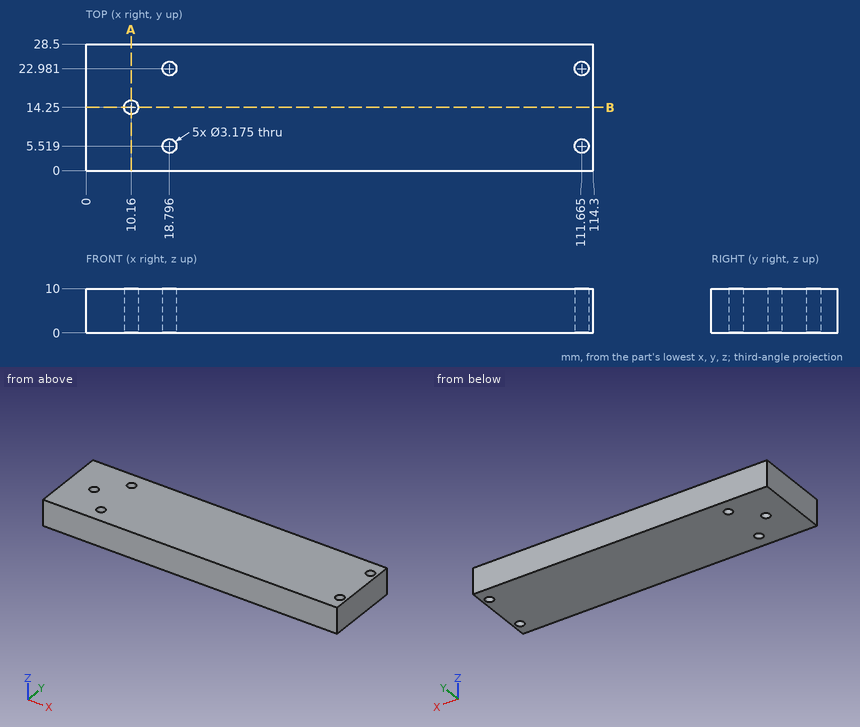
Geometry: see drawing. Coordinates: mm, zero at the bounding-box minimum. Give positions to 0.01 mm unless a question says otherwise; leave off trailing zeros. Order: outer loops, then holes, each group sorted by start corner. A loop starts at its lowest first (then second) coordinate and runs counter-clockwise, first axis right, second up. Notation, with made-up numbers: M -38,-23.5 L -14,-23.5 A19 cw -14,7.5 Z; hole C 60,61 d9. An arc over 180 degrees is marked long. Answer as a JSON object with one key per item and string values.
1. Cut plane B-B, the plane y = 14.25. Output: boundary loops of the cut face in (x, z).
Result sheet:
{"outline": "M 0,0 L 8.57,0 L 8.57,10 L 0,10 Z; M 11.75,0 L 114.3,0 L 114.3,10 L 11.75,10 Z"}
2. Ray query, line 1 (X direction, y = 5.5, z = 1.5); line 2 (X direction, y = 22.25, z = 6.5) (1 decimal); line 3 (X direction, y = 14.5, z = 8.5). Return the intervals inside material, ascending. Write a range as [from, to].
Result sheet:
{"line 1": "[0, 17.21], [20.38, 110.08], [113.25, 114.3]", "line 2": "[0, 17.4], [20.2, 110.3], [113.1, 114.3]", "line 3": "[0, 8.59], [11.73, 114.3]"}
3. Cut plane A-A, the plane x = 10.16. Output: boundary loops of the cut face in (y, z).
Result sheet:
{"outline": "M 0,0 L 12.66,0 L 12.66,10 L 0,10 Z; M 15.84,0 L 28.5,0 L 28.5,10 L 15.84,10 Z"}
